Geometry: final body of the model. Coordinates: model frame, mm. Round coordinates to 2 decimals unless told otherwise and drop trailing zeros. Loops run counter-clockwise (first coordinate to the right, second up) from the corner with the lowest first, then second, coordinate; pieces in that order, holes last. Notation, with made-up numbers: M -36,2.5 L 5,2.5 A25 ccw 5,18.5 Z; hole C 6.5,-39.5 d5. An arc over 180 degrees is marked long. Answer as a JSON object with one key per item and string values.
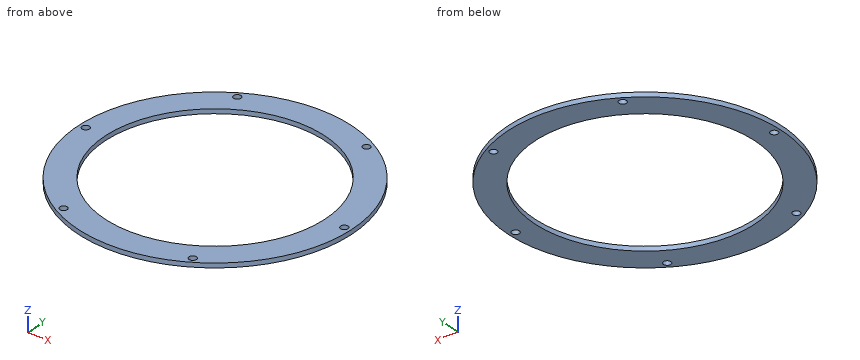
```python
from build123d import *

# Parameters (mm, degrees)
STATOR_CLAMP_START  = 20
SKETCH_1_R          = 61
SKETCH_1_R_2        = 49
STATOR_CLAMP_DEPTH  = 2
SKETCH_2_R          = 1.65
THROUGH_HOLES_DEPTH = 100


with BuildPart() as part:
    # Эскиз1 → Stator_clamp (new body)
    with BuildSketch(Plane.XY.offset(STATOR_CLAMP_START)):
        Circle(SKETCH_1_R)
        Circle(SKETCH_1_R_2, mode=Mode.SUBTRACT)
    extrude(amount=STATOR_CLAMP_DEPTH)

    # Эскиз2 → Through_holes (cut, symmetric)
    with BuildSketch(Plane.XY):
        with Locations((58, 0)):
            Circle(SKETCH_2_R)
        with Locations((29, 50.229473419)):
            Circle(SKETCH_2_R)
        with Locations((-29, 50.229473419)):
            Circle(SKETCH_2_R)
        with Locations((-58, 0)):
            Circle(SKETCH_2_R)
        with Locations((-29, -50.229473419)):
            Circle(SKETCH_2_R)
        with Locations((29, -50.229473419)):
            Circle(SKETCH_2_R)
    extrude(amount=THROUGH_HOLES_DEPTH, both=True, mode=Mode.SUBTRACT)


solid = part.part
```
1) Cut plane B-B on x = 16. Return the cut outline in (y, z), and give its area (3 significant figures).
Geometry results:
{"outline": "M -58.86,20 L -46.31,20 L -46.31,22 L -58.86,22 Z; M 46.31,20 L 58.86,20 L 58.86,22 L 46.31,22 Z", "area": "50.2 mm2"}
2) Cut plane A-A on y = 0. Return the cut outline in (x, z).
Geometry results:
{"outline": "M -61,20 L -59.65,20 L -59.65,22 L -61,22 Z; M -56.35,20 L -49,20 L -49,22 L -56.35,22 Z; M 49,20 L 56.35,20 L 56.35,22 L 49,22 Z; M 59.65,20 L 61,20 L 61,22 L 59.65,22 Z"}
3) Cut plane C-C on x = 29. Return the cut outline in (y, z).
Geometry results:
{"outline": "M -53.67,20 L -51.88,20 L -51.88,22 L -53.67,22 Z; M -48.58,20 L -39.5,20 L -39.5,22 L -48.58,22 Z; M 39.5,20 L 48.58,20 L 48.58,22 L 39.5,22 Z; M 51.88,20 L 53.67,20 L 53.67,22 L 51.88,22 Z"}
4) Cut plane D-D on y = 22.5. Return the cut outline in (x, z), and give its area (3 significant figures).
Geometry results:
{"outline": "M -56.7,20 L -43.53,20 L -43.53,22 L -56.7,22 Z; M 43.53,20 L 56.7,20 L 56.7,22 L 43.53,22 Z", "area": "52.7 mm2"}
5) Line query: probe 1 along Y at (x, z) = (-29, 20.6); probe 2 along X at (y, z) = (-1, 21.85); probe 3 along Y at (x, z) = (0, 21). Output: solid intervals per line, ascending.
Geometry results:
{"probe 1": "-53.67 to -51.88, -48.58 to -39.5, 39.5 to 48.58, 51.88 to 53.67", "probe 2": "-60.99 to -59.31, -56.69 to -48.99, 48.99 to 56.69, 59.31 to 60.99", "probe 3": "-61 to -49, 49 to 61"}
